Input: part model. Units: mm. Frame: model coordinates. Face numbers are marked on the shaded views. Coordinates: 2 decimals unless noted, no trailing zeros. Order: outer loops, then holes, each group sorted by start corner. A loop starts at its lowest first (then second) coordinate and runs counter-clockwise, first axis right, second up.
from build123d import *

# Parameters (mm, degrees)
ESQUISSE1_R      = 13.5
ESQUISSE1_R_2    = 11
EXTRUSION1_DEPTH = 111
CHANFREIN1_SIZE  = 2.5
CHANFREIN1_SIZE2 = 0.5
CHANFREIN2_SIZE  = 2.5
CHANFREIN2_SIZE2 = 0.5


with BuildPart() as part:
    # Esquisse1 → Extrusion1 (new body, symmetric)
    with BuildSketch(Plane(origin=(0, 0, 0), x_dir=(1, 0, 0), z_dir=(0, 1, 0))):
        with Locations(Location((0, 0, 0), (0, 0, 270))):  # turned: the seam where the file's is
            Circle(ESQUISSE1_R)
        with Locations(Location((0, 0, 0), (0, 0, 270))):  # turned: the seam where the file's is
            Circle(ESQUISSE1_R_2, mode=Mode.SUBTRACT)
    extrude(amount=EXTRUSION1_DEPTH, both=True)

    # Chanfrein1
    chanfrein1_edges = [part.edges().sort_by_distance(p)[0] for p in [
        (0, -111, -13.5),
    ]]
    chanfrein1_side = [part.faces().sort_by_distance(p)[0] for p in [
        (0, 0, -13.5),
    ]]
    chamfer(chanfrein1_edges, length=CHANFREIN1_SIZE, length2=CHANFREIN1_SIZE2, reference=chanfrein1_side[0])

    # Chanfrein2
    chanfrein2_edges = [part.edges().sort_by_distance(p)[0] for p in [
        (0, 111, -13.5),
    ]]
    chanfrein2_side = [part.faces().sort_by_distance(p)[0] for p in [
        (0, 1.25, -13.5),
    ]]
    chamfer(chanfrein2_edges, length=CHANFREIN2_SIZE, length2=CHANFREIN2_SIZE2, reference=chanfrein2_side[0])


solid = part.part
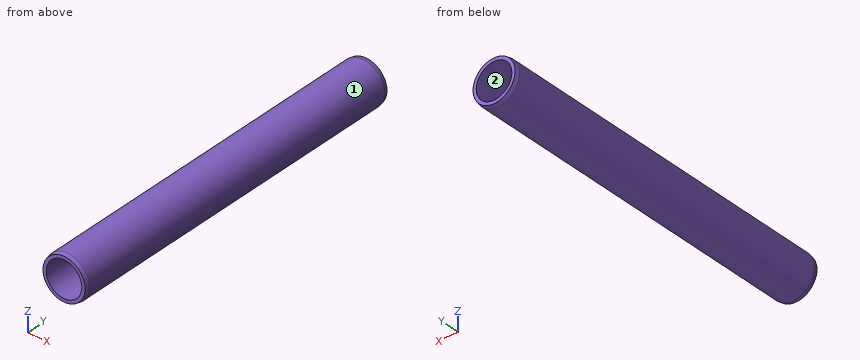
Item 1: Pin query (flat end, axial travel): pin 1 Ø2 at (x, y) = (-9, -38.5) entering from +Z; pin 2 Ø6 at (y, z) = (56.5, -5) entering from +X; pin 3 Ø1.5 at (y, z) = (44, -9) entering from +X. Return the tip coordinate at first contact, or that it passes through.
Response values:
pin 1: stops at z = 10.87
pin 2: stops at x = 13.35
pin 3: stops at x = 10.69
Item 2: Cut plane C-C on y = -93.5. Return loops of the section in (x, z).
Response values:
outline: circle Ø27 at (0, 0); hole circle Ø22 at (0, 0)
Item 3: Ray query, probe 1 along X at (y, z) = (-64, 0); probe 2 along Z at (x, y) = (2.75, 46); probe 3 along Z at (x, y) = (4, 90). Return the intervals inside material, ascending.
Response values:
probe 1: x = -13.5 to -11, 11 to 13.5
probe 2: z = -13.22 to -10.65, 10.65 to 13.22
probe 3: z = -12.89 to -10.25, 10.25 to 12.89
Item 4: Cut plane A-A on z = 0. Return loops of the section in (x, y), then the cut area to 3 significant figures.
Response values:
outline: (-13.5, -108.5) - (-13, -111) - (-11, -111) - (-11, 111) - (-13, 111) - (-13.5, 108.5) - close; (11, -111) - (13, -111) - (13.5, -108.5) - (13.5, 108.5) - (13, 111) - (11, 111) - close
area: 1,110 mm2
Item 5: Draft query along X for the marked faces 1 and 2. Return one class per face: pulls with the +X half, pulls with the -X half, needs draft (parallel to the pull), parting line crosses it, or undercut.
Response values:
face 1: parting line crosses it
face 2: undercut
Item 6: Cut plane B-B on x = 0. Return loops of the section in (y, z), then the cut area to 3 significant figures.
Response values:
outline: (-111, -13) - (-108.5, -13.5) - (108.5, -13.5) - (111, -13) - (111, -11) - (-111, -11) - close; (-111, 11) - (111, 11) - (111, 13) - (108.5, 13.5) - (-108.5, 13.5) - (-111, 13) - close
area: 1,110 mm2
